Could you check a few things on this model? Use its own coordinates, in mm. Face numbers are marked on the shaded views. A direction names the side the tool comes from. Round coordinates to 2 decimals unless told otherwise and drop trailing zeros. Loops run counter-clockwise (first coordinate to the right, second up) from the corner with the lowest first, then second, coordinate; pieces in that order, holes last. Notation, with made-up numbers: (58, 77.5) -> (116, 77.5) arc R15 ccw to (116, 93.5) -> close; hole circle Ø7 at (14, -21.5). An arc over 180 degrees is marked (long way). Write each question's results on one line, items separated by ' | '.
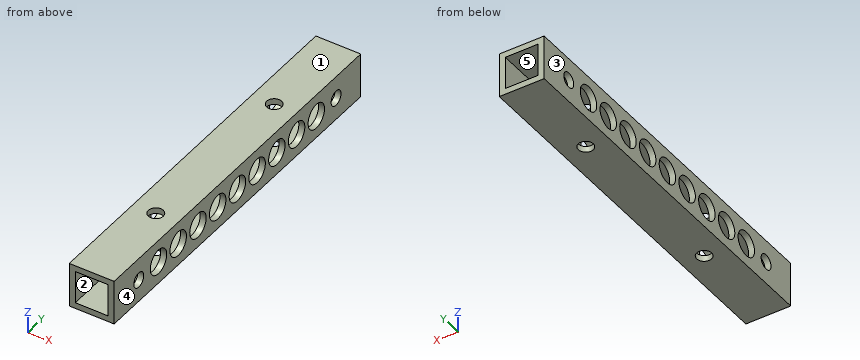
Autodesk Inventor part; units mm, degrees
ref_plane "YZ Plane" through (0, 0, 0) normal (1, 0, 0) x (0, 1, 0)
ref_plane "XZ Plane" through (0, 0, 0) normal (0, 1, 0) x (-1, 0, 0)
ref_plane "XY Plane" through (0, 0, 0) normal (0, 0, 1) x (1, 0, 0)
sketch "スケッチ1" plane through (0, 0, 0) normal (0, 1, 0) x (-1, 0, 0)
  line L0 (0, 0) -> (9, 0)
  line L1 (9, 0) -> (9, -9)
  line L2 (9, -9) -> (0, -9)
  line L3 (0, -9) -> (0, 0)
  line L4 (1.2, -1.2) -> (7.8, -1.2)
  line L5 (7.8, -1.2) -> (7.8, -7.8)
  line L6 (7.8, -7.8) -> (1.2, -7.8)
  line L7 (1.2, -7.8) -> (1.2, -1.2)
  dimension "d0" = 9
  dimension "d1" = 9
  dimension "d2" = 6.6
  dimension "d3" = 6.6
  dimension "d4" = 1.2
  dimension "d5" = 1.2
extrude "押し出し1" add sketch "スケッチ1" along normal blind 75
sketch "スケッチ2" plane through (-9, 0, -9) normal (-1, 0, 0) x (0, 0, 1)
  line L0 (0, 0) -> (9, 0)
  line L1 (0, 75) -> (9, 75)
  line L2 (0, 0) -> (0, 75)
  point P0 (4.5, 7.5)
  point P1 (4.5, 67.5)
  dimension "d8" = 7.5
  dimension "d9" = 7.5
  dimension "d10" = 4.5
  dimension "d11" = 4.5
hole "穴1" at (-9, 7.5, -4.5) at (-9, 67.5, -4.5) direction (1, 0, 0) diameter 3 end through all
sketch "スケッチ3" plane through (0, 0, -9) normal (0, 0, -1) x (-1, 0, 0)
  line L0 (9, 0) -> (9, 75)
  line L1 (0, 75) -> (9, 75)
  line L2 (0, 0) -> (9, 0)
  point P0 (4.5, 19.5)
  point P1 (4.5, 55.5)
  dimension "d19" = 4.5
  dimension "d20" = 4.5
  dimension "d21" = 19.5
  dimension "d22" = 19.5
hole "穴2" at (-4.5, 19.5, -9) at (-4.5, 55.5, -9) direction (0, 0, 1) diameter 3 end through all
sketch "スケッチ4" plane through (-9, 0, -9) normal (-1, 0, 0) x (0, 0, 1)
  circle A0 centre (4.5, 67.5) radius 1.5
  circle A1 centre (4.5, 7.5) radius 1.5
  line L0 (4.5, 67.5) -> (4.5, 7.5)
  point P0 (9, 0)
  point P1 (4.5, 61.5)
  point P2 (4.5, 55.5)
  point P3 (4.5, 49.5)
  point P4 (4.5, 43.5)
  point P5 (4.5, 37.5)
  point P6 (4.5, 31.5)
  point P7 (4.5, 25.5)
  point P8 (4.5, 19.5)
  point P9 (4.5, 13.5)
  dimension "d30" = 60
  dimension "d31" = 6
  dimension "d34" = 6
hole "穴3" at (-9, 61.5, -4.5) at (-9, 55.5, -4.5) at (-9, 49.5, -4.5) at (-9, 43.5, -4.5) at (-9, 37.5, -4.5) at (-9, 31.5, -4.5) at (-9, 25.5, -4.5) at (-9, 19.5, -4.5) at (-9, 13.5, -4.5) direction (1, 0, 0) diameter 5 end through all
equation "\"d1\" = d0"
equation "\"d3\" = d2"
properties part number "前後直動12x12_2" material "アルミニウム 6061"
1) I want a section at C-C, the plane y = 7.5. Write out the boundary of the cut face in (x, z).
Model answer:
outline: (-9, -9) -> (0, -9) -> (0, -6) -> (-1.2, -6) -> (-1.2, -7.8) -> (-7.8, -7.8) -> (-7.8, -6) -> (-9, -6) -> close; (-9, -3) -> (-7.8, -3) -> (-7.8, -1.2) -> (-1.2, -1.2) -> (-1.2, -3) -> (0, -3) -> (0, 0) -> (-9, 0) -> close
2) I want a section at A-A, the plane y = 55.5. Write out the boundary of the cut face in (x, z).
Model answer:
outline: (-9, -9) -> (-6, -9) -> (-6, -7.8) -> (-7.8, -7.8) -> (-7.8, -7) -> (-9, -7) -> close; (-9, -2) -> (-7.8, -2) -> (-7.8, -1.2) -> (-6, -1.2) -> (-6, 0) -> (-9, 0) -> close; (-3, -9) -> (0, -9) -> (0, -7) -> (-1.2, -7) -> (-1.2, -7.8) -> (-3, -7.8) -> close; (-3, -1.2) -> (-1.2, -1.2) -> (-1.2, -2) -> (0, -2) -> (0, 0) -> (-3, 0) -> close
3) I need wall thicknesses on line 1 (X direction, y = 43, z = -7.25); line 2 (Z direction, x = -0.6, y = 61.5). Which ranges of each line are inside material? Lowest first, please.
Model answer:
line 1: x = -9 to -7.8, -1.2 to 0 | line 2: z = -9 to -7, -2 to 0
4) I want a section at D-D, the plane z = -4. Give the number of separate pieces and of enclosed holes in the cut face, plus the area to 3 significant figures.
Model answer:
separate pieces: 24 | enclosed holes: 0 | area: 60.6 mm2
5) For the marked faces 4 and 5, which set-ups out of +Z, -Z, +X, -X, +Y, -Y let a thin tool reach every point of the face, with its end or its side?
Model answer:
face 4: +Z, -Z, +X, +Y, -Y | face 5: +Y, -Y
6) If we mould it in two halves opening along X, with no side actions, what happens to the marked faces 1, 2 and 3? For each: released by +X, released by -X, zero draft, split by the parting line, or undercut.
Model answer:
face 1: zero draft | face 2: undercut | face 3: released by -X
7) I want a section at B-B, the plane x = -4.5. Write out the boundary of the cut face in (y, z).
Model answer:
outline: (0, -9) -> (18, -9) -> (18, -7.8) -> (0, -7.8) -> close; (0, -1.2) -> (18, -1.2) -> (18, 0) -> (0, 0) -> close; (21, -9) -> (54, -9) -> (54, -7.8) -> (21, -7.8) -> close; (21, -1.2) -> (54, -1.2) -> (54, 0) -> (21, 0) -> close; (57, -9) -> (75, -9) -> (75, -7.8) -> (57, -7.8) -> close; (57, -1.2) -> (75, -1.2) -> (75, 0) -> (57, 0) -> close
